from build123d import *

# Parameters (mm, degrees)
CROQUIS3_W            = 27.632411408
CROQUIS3_H            = 25
CROQUIS5_R            = 11.25
CORTAR_EXTRUIR1_DEPTH = 45.872599214
CROQUIS6_R            = 21
CORTAR_EXTRUIR2_DEPTH = 3


with BuildPart() as part:
    # Croquis3 → Revolución5 (revolve)
    with BuildSketch(Plane(origin=(0, 0, 0), x_dir=(0, 0, -1), z_dir=(1, 0, 0)), mode=Mode.PRIVATE) as revoluci_n5_sk:
        with Locations((13.816205704, -12.5)):
            Rectangle(CROQUIS3_W, CROQUIS3_H)
    revolve(revoluci_n5_sk.sketch.rotate(Axis((0, 0, 45.885013439), (0, 0, -1)), 270), axis=Axis((0, 0, 45.885013439), (0, 0, -1)))

    # Croquis5 → Cortar-Extruir1 (cut, through all)
    with BuildSketch(Plane.XY):
        Circle(CROQUIS5_R)
    extrude(amount=-CORTAR_EXTRUIR1_DEPTH, mode=Mode.SUBTRACT)

    # Croquis6 → Cortar-Extruir2 (cut)
    with BuildSketch(Plane.XY):
        Circle(CROQUIS6_R)
    extrude(amount=-CORTAR_EXTRUIR2_DEPTH, mode=Mode.SUBTRACT)


solid = part.part
Check sheet for the modelled part. Datum: model origin and axes. Units: mm. A direction names the side the tool comes from. Give positions to 0.01 mm unless a question says otherwise; leave off trailing zeros. Order: outer loops, then holes, each group sorted by start corner. A loop starts at its lowest first (then second) coordinate and runs counter-clockwise, first axis right, second up. Notation, with made-up numbers: (14.5, 43.5) - (61.5, 43.5) arc R7 ccw to (61.5, 52.5) - close; hole circle Ø10 at (38.25, -5). An arc over 180 degrees is marked (long way). Answer as CSV lines item,"result".
1. Go/stop test with flat-tipped pins: P1, Ø1.5, axis at x = 1.5, z = -7, coming from the +Y side; P2, Ø6, axis at x = -17, z = -12, coming from the -Y side; P3, Ø12, axis at x = -13, z = -4.5, coming from the +Y side. Record where each tip stops, or that it passes through.
Result sheet:
P1,"y = 24.99"
P2,"y = -20.71"
P3,"y = 24"
2. Mould release check, pull along Y, two halves, no side actions. Record for faces 3 (the face through (5.19, -9.98, -15.14)), 4 (the face through (-5.7, -20.5, 0)), 5 (the face through (23.846, -7.509, -14.01)): released by +Y, released by -Y, zero draft, split by the parting line, or undercut.
Result sheet:
face 3,"undercut"
face 4,"zero draft"
face 5,"split by the parting line"
3. Section check D-D (z = -16.75). Record the boundary of the cut face in (x, y).
Result sheet:
outline,"circle Ø50 at (0, 0); hole circle Ø22.5 at (0, 0)"
4. Scan lines: probe 1 along Y at (x, z) = (0, -17); probe 2 along Y at (x, z) = (0, -1.7); probe 3 along Z at (x, y) = (5.5, 18). Record each from-to range of solid material in increasing order. Write a range as from..to.
Result sheet:
probe 1,"-25..-11.25, 11.25..25"
probe 2,"-25..-21, 21..25"
probe 3,"-27.63..-3"
5. Section check C-C (x = -15). Record the boundary of the cut face in (y, z).
Result sheet:
outline,"(-20, -27.63) - (20, -27.63) - (20, 0) - (14.7, 0) - (14.7, -3) - (-14.7, -3) - (-14.7, 0) - (-20, 0) - close"
6. Tool access check on faces 1 (the face through (9, -9, -3)), 2 (the face through (11, 5, -27.632)). Record the directions out of +Z, -Z, +X, -X, +Y, -Y that give a thin tool (end or side, any length) a straight path to the whole face; none if there is none.
Result sheet:
face 1,"+Z"
face 2,"-Z, +X, -X, +Y, -Y"
7. Section check A-A (x = 0). Record the boundary of the cut face in (y, z), then the cut area to 3 significant figures.
Result sheet:
outline,"(-25, -27.63) - (-11.25, -27.63) - (-11.25, -3) - (-21, -3) - (-21, 0) - (-25, 0) - close; (11.25, -27.63) - (25, -27.63) - (25, 0) - (21, 0) - (21, -3) - (11.25, -3) - close"
area,"701 mm²"
